```python
from build123d import *

# Parameters (mm, degrees)
SKETCH8_W               = 74
SKETCH8_H               = 10
BOSS_EXTRUDE9_DEPTH     = 46
FILLET8_R               = 12
FILLET9_R               = 12
CUT_EXTRUDE3_DEPTH      = 88.704047797
CUT_EXTRUDE3_DEPTH_BACK = 88.704047797
SKETCH13_R              = 6
BOSS_EXTRUDE10_DEPTH    = 14
CUT_EXTRUDE4_REACH      = 99.719
SKETCH15_W              = 5
SKETCH15_H              = 52
SKETCH26_R              = 16
BOSS_EXTRUDE11_DEPTH    = 14
FILLET11_R              = 5
FILLET12_START          = 5
FILLET12_DEPTH          = 14
FILLET12_START_2        = -27.782193151
FILLET12_2_DEPTH        = 64.0000001
SKETCH28_R              = 6
CUT_EXTRUDE5_DEPTH      = 92.863527091
RIB2_REACH              = 92.05
SKETCH31_WALL_W         = 233.324966138
SKETCH31_WALL_H         = 10
FILLET13_R              = 5
SKETCH36_R              = 6
CUT_EXTRUDE6_DEPTH      = 92.863527091


with BuildPart() as part:
    # Sketch8 → Boss-Extrude9 (new body)
    with BuildSketch(Plane.XY):
        with Locations((4.217806949, -5)):
            Rectangle(SKETCH8_W, SKETCH8_H)
    extrude(amount=BOSS_EXTRUDE9_DEPTH)

    # Fillet8
    fillet8_edges = [part.edges().sort_by_distance(p)[0] for p in [
        (-32.782193051, -5, 46),
    ]]
    fillet(fillet8_edges, radius=FILLET8_R)

    # Fillet9
    fillet9_edges = [part.edges().sort_by_distance(p)[0] for p in [
        (41.217806949, -5, 46),
    ]]
    fillet(fillet9_edges, radius=FILLET9_R)

    # Sketch10 → Cut-Extrude3 (cut, two sides: drawn at the far end of the back side and taken through both)
    with BuildSketch(Plane.ZY.offset(32.782193051).offset(-CUT_EXTRUDE3_DEPTH_BACK)):
        with BuildLine():
            Line((5, 102.54188241), (5, 0))
            ThreePointArc((5, 0), (3.535533906, -3.535533906), (0, -5))
            Line((0, -5), (-102.54188241, -5))
            Line((-102.54188241, -5), (-247.558003226, 140.016120816))
            Line((-247.558003226, 140.016120816), (-140.016120816, 247.558003226))
            Line((-140.016120816, 247.558003226), (5, 102.54188241))
        make_face()
    extrude(amount=CUT_EXTRUDE3_DEPTH + CUT_EXTRUDE3_DEPTH_BACK, mode=Mode.SUBTRACT)

    # Sketch13 → Boss-Extrude10 (add)
    with BuildSketch(Plane.XY):
        with BuildLine():
            Line((-11.782193051, 0), (20.217806949, 0))
            Line((20.217806949, 0), (20.217806949, 52))
            ThreePointArc((20.217806949, 52), (4.217806949, 68), (-11.782193051, 52))
            Line((-11.782193051, 52), (-11.782193051, 0))
        make_face()
        with Locations((4.217806949, 52)):
            Circle(SKETCH13_R, mode=Mode.SUBTRACT)
    extrude(amount=BOSS_EXTRUDE10_DEPTH)

    # Sketch15 → Cut-Extrude4 (cut, up to next)
    with BuildSketch(Plane.ZY.offset(11.782193051), mode=Mode.PRIVATE) as cut_extrude4_sk1:
        with Locations((2.5, 26)):
            Rectangle(SKETCH15_W, SKETCH15_H)
    cut_extrude4_tool1 = extrude(cut_extrude4_sk1.sketch, amount=-CUT_EXTRUDE4_REACH, mode=Mode.PRIVATE) & part.part
    add(cut_extrude4_tool1.solids().sort_by_distance((-11.782193, 26, 2.5))[0], mode=Mode.SUBTRACT)

    # Sketch26 → Boss-Extrude11 (add)
    with BuildSketch(Plane(origin=(0, 0, 0), x_dir=(-1, 0, 0), z_dir=(0, 0, -1))):
        with Locations((-4.217806949, 52)):
            Circle(SKETCH26_R)
    extrude(amount=-BOSS_EXTRUDE11_DEPTH)

    # Fillet11
    fillet11_edges = [part.edges().sort_by_distance(p)[0] for p in [
        (4.217806949, 0, 14),
    ]]
    fillet(fillet11_edges, radius=FILLET11_R)

    # Fillet12: read off the stored shape, not the designer's step
    # Fillet12 outline → Fillet12 (add)
    with BuildSketch(Plane.XY.offset(FILLET12_START)):
        with BuildLine():
            Line((-11.782193051, 0), (-11.782193051, 16))
            ThreePointArc((-11.782193051, 16), (-16.468484552, 4.686291501), (-27.782193051, 0))
            Line((-27.782193051, 0), (-11.782193051, 0))
        make_face()
        with BuildLine():
            Line((20.217806949, 16), (20.217806949, 0))
            Line((20.217806949, 0), (36.217806949, 0))
            ThreePointArc((36.217806949, 0), (24.90409845, 4.686291501), (20.217806949, 16))
        make_face()
    extrude(amount=FILLET12_DEPTH)

    # Fillet12 2 outline → Fillet12 2 (cut)
    with BuildSketch(Plane.YZ.offset(FILLET12_START_2)):
        with BuildLine():
            Line((16, 19), (0, 19))
            ThreePointArc((0, 19), (1.464466094, 15.464466094), (5, 14))
            Line((5, 14), (16, 14))
            Line((16, 14), (16, 19))
        make_face()
    extrude(amount=FILLET12_2_DEPTH, mode=Mode.SUBTRACT)

    # Sketch28 → Cut-Extrude5 (cut, through all)
    with BuildSketch(Plane(origin=(0, 0, 0), x_dir=(-1, 0, 0), z_dir=(0, 0, -1))):
        with Locations((-4.217806949, 52)):
            Circle(SKETCH28_R)
    extrude(amount=-CUT_EXTRUDE5_DEPTH, mode=Mode.SUBTRACT)

    # Sketch31 wall → Rib2 (add, up to next)
    with BuildSketch(Plane(origin=(4.217806949, 20, 30), x_dir=(0, -0.780868809443, 0.624695047554), z_dir=(0, 0.624695047554, 0.780868809443)), mode=Mode.PRIVATE) as rib2_sk1:
        Rectangle(SKETCH31_WALL_W, SKETCH31_WALL_H)
    rib2_tool1 = extrude(rib2_sk1.sketch, amount=-RIB2_REACH, mode=Mode.PRIVATE) - part.part
    add(rib2_tool1.solids().sort_by_distance((4.217806949, 20, 30))[0])

    # Fillet13
    fillet13_edges = [part.edges().sort_by_distance(p)[0] for p in [
        (-0.782193051, 0, 32.5),
        (-0.782193051, 1.464466094, 15.464466094),
        (-0.782193051, 22.5, 14),
        (9.217806949, 1.464466094, 15.464466094),
        (9.217806949, 22.5, 14),
        (9.217806949, 0, 32.5),
    ]]
    fillet(fillet13_edges, radius=FILLET13_R)

    # Sketch36 → Cut-Extrude6 (cut, through all)
    with BuildSketch(Plane(origin=(0, 0, 0), x_dir=(1, 0, 0), z_dir=(0, 1, 0))):
        with Locations(Location((-20.782193051, -34, 0), (0, 0, 270))):
            Circle(SKETCH36_R)
        with Locations(Location((29.217806949, -34, 0), (0, 0, 270))):
            Circle(SKETCH36_R)
    extrude(amount=-CUT_EXTRUDE6_DEPTH, mode=Mode.SUBTRACT)


solid = part.part
```
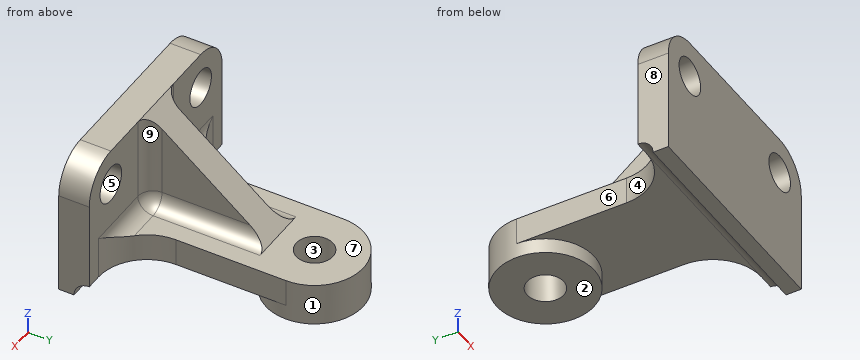
Build history of the part. All positions in model axes, mm. Face numbers are marked on the shaded views. A direction names the side the tool comes from. Give positions to 0.01 mm unless a question says otherwise; leave off trailing zeros. Order: outer loops, then holes, each group sorted by start corner. A loop starts at its lowest first (then second) coordinate and runs counter-clockwise, first axis right, second up. Notation, with made-up numbers: M 49,-10.75 L 100,-10.75 A21 cw 100,13.25 Z; hole C 32,16 d1. An arc over 180 degrees is marked long. Write item = value, one per line. Start each with the question number.
(1) Slice it at A-A on y = 28.5. Write the cut outline in (x, z), plus the area to 3 significant figures.
(2) Slice it at C-C on z = 33. Write the cut outline in (x, y), plus the area to 3 significant figures.
(3) Which spindle directions (+Z, -Z, +X, -X, +Y, -Y) get a long thin tool onto all of the face, cutting with end or side? Do the marked faces 5, 6, 7, 8 and 9. Say none if no direction does.
(4) Two-plate mould, pull along Y, no slides. Class the marked faces 1, 2, 3 and 4: released by +Y, released by -Y, zero draft, split by the parting line, or undercut.
(5) Probe L1, parallel to X at y = -6.5, z = 34; L2, parallel to Z at x = 19.5, y = 22.5; L3, parallel to X at y = 31.5, z = 7.5. List the from-to ranges inside material, lowest first. Write a range as [from, to].
(6) Slice it at B-B on x = -24.5. Write the cut outline in (y, z).
(7) Pin check, flat tips, straight feed: pin 1 Ø7 at (x, z) = (29.22, 34) entering from +Y; pin 2 Ø8 at (x, z) = (-23.5, 28) entering from +Y; pin 3 Ø1 at (y, z) = (2, 29) entering from -X; pin 4 Ø10 at (y, z) = (34, 9.5) entering from +X. Stop position of each tip, or through.
Responses:
q1.outline = M -11.78,5 L 20.22,5 L 20.22,14 L 14.22,14 A5 cw 9.22,19 L 9.22,23.2 L -0.78,23.2 L -0.78,19 A5 cw -5.78,14 L -11.78,14 Z
q1.area = 391 mm2
q2.outline = M -32.78,-10 L -26.7,-10 L -26.7,0 L -32.78,0 Z; M -14.87,-10 L 23.3,-10 L 23.3,0 L 14.22,0 A5 cw 9.22,5 L 9.22,16.25 L -0.78,16.25 L -0.78,5 A5 cw -5.78,0 L -14.87,0 Z; M 35.13,-10 L 41.22,-10 L 41.22,0 L 35.13,0 Z
q2.area = 677 mm2
q3.face_5 = +Y, -Y
q3.face_6 = +Z, -Z, -X, +Y
q3.face_7 = +Z, +Y
q3.face_8 = +Z, -Z, -X, +Y, -Y
q3.face_9 = +Z, +X, +Y
q4.face_1 = undercut
q4.face_2 = zero draft
q4.face_3 = undercut
q4.face_4 = released by +Y
q5.L1 = [-32.78, -26.78], [-14.78, 23.22], [35.22, 41.22]
q5.L2 = [5, 14]
q5.L3 = [-11.78, 20.22]
q6.outline = M -10,0 L -5,0 A5 cw 0,5 L 0.34,5 L 0.34,17.19 A5 cw 0,19 L 0,29.29 L -10,29.29 Z; M -10,38.71 L 0,38.71 L 0,45.41 L -10,45.41 Z
q7.pin_1 = through
q7.pin_2 = 0
q7.pin_3 = -2.21
q7.pin_4 = 20.22
